from build123d import *

# Parameters (mm, degrees)
SKETCH1_R           = 5.75
SKETCH1_R_2         = 3
BOSS_EXTRUDE1_DEPTH = 6
SKETCH1_3_R         = 5.75
SKETCH1_3_R_2       = 3
BOSS_EXTRUDE2_DEPTH = 12


with BuildPart() as part:
    # Sketch1 → Boss-Extrude1 (new body)
    with BuildSketch(Plane.XY):
        Polygon((-3.464101615, 6), (-6.92820323, 0), (-3.464101615, -6), (3.464101615, -6), (6.92820323, 0), (3.464101615, 6), align=None)
        Circle(SKETCH1_R, mode=Mode.SUBTRACT)
        Circle(SKETCH1_R)
        Circle(SKETCH1_R_2, mode=Mode.SUBTRACT)
        Circle(SKETCH1_R_2)
    extrude(amount=BOSS_EXTRUDE1_DEPTH)

    # Sketch1_3 → Boss-Extrude2 (add)
    with BuildSketch(Plane.XY):
        Circle(SKETCH1_3_R)
        Circle(SKETCH1_3_R_2, mode=Mode.SUBTRACT)
    extrude(amount=-BOSS_EXTRUDE2_DEPTH)


solid = part.part
Input: part model. Units: mm. Frame: model coordinates. A direction names the side the tool comes from. Coordinates: 2 decimals unless noted, no trailing zeros. Loops run counter-clockwise (first coordinate to the right, second up) from the corner with the lowest first, then second, coordinate; pieces in that order, holes last. Notation, with made-up numbers: (65.25, 46) - (73.25, 46) arc R16 cw to (73.25, 62) - close; hole circle Ø5 at (26.5, 74.5). An arc over 180 degrees is marked (long way). Answer in a Markdown table with one row per item. Add a question column.
Item 1: Contact query for flat-ended pins moving along their axis: P1, Ø4, axis at y = -1.5, z = -7.5, coming from the -X side; P2, Ø1.5, axis at x = -2, z = -4, coming from the +Y side; P3, Ø1.5, axis at x = -4, z = -5, coming from the -Y side; P4, Ø5, axis at x = 0.5, y = -1, coming from the -Z side. Output: stop coordinate, or through.
Item 2: Section query B-B on x = 0. Return the cut outline in (y, z), then the cut area to 3 significant figures.
Item 3: Section query D-D on z = -1.5. Return the cut outline in (x, y), then the cut area to 3 significant figures.
Item 4: Section query C-C on y = 3.5. Return the cut outline in (x, z).
Item 5: Section query A-A on z = 2. Return the cut outline in (x, y).
Item 6: Mould query, pull axis X, two halves, no side actions, for faces 3 (the cylindrical face through (-3, 0, -6)), 4 (the flat face through (0, 0, 0)), 5 (the flat face through (0, -6, 3)), 6 (the flat face through (-5.22, -2.96, 2.96)). Classes: released by +X, released by -X, zero draft, split by the parting line, or undercut.
Item 7: Access query for faces 1 (the flat face through (6, 1, 0)), 2 (the flat face through (2.5, -2.5, -12)). Directions: +Z, -Z, +X, -X, +Y, -Y. A direction counts if a zero-diameter tool reaches every point of the face in a straight line with its end or side. Return the directions, or none.
Item 8: Line query: line 1 along Y through (x, z) = (0, -5.25); line 2 along Z through (x, y) = (1.5, 0.5); line 3 along Y through (x, z) = (2.5, -7.5). Output: solid intervals per line, ascending. Write a range as [from, to].
Recorded:
| question | item | result |
|---|---|---|
| 1 | P1 | x = -5.75 |
| 1 | P2 | y = 5.61 |
| 1 | P3 | y = -4.74 |
| 1 | P4 | z = -12 |
| 2 | outline | (-6, 0) - (-5.75, 0) - (-5.75, -12) - (-3, -12) - (-3, 0) - (3, 0) - (3, -12) - (5.75, -12) - (5.75, 0) - (6, 0) - (6, 6) - (-6, 6) - close |
| 2 | area | 138 mm^2 |
| 3 | outline | circle Ø11.5 at (0, 0); hole circle Ø6 at (0, 0) |
| 3 | area | 75.6 mm^2 |
| 4 | outline | (-4.91, 0) - (-4.56, 0) - (-4.56, -12) - (4.56, -12) - (4.56, 0) - (4.91, 0) - (4.91, 6) - (-4.91, 6) - close |
| 5 | outline | (-6.93, 0) - (-3.46, -6) - (3.46, -6) - (6.93, 0) - (3.46, 6) - (-3.46, 6) - close |
| 6 | face 3 | undercut |
| 6 | face 4 | undercut |
| 6 | face 5 | zero draft |
| 6 | face 6 | released by -X |
| 7 | face 1 | -Z |
| 7 | face 2 | -Z, +X, -X, +Y, -Y |
| 8 | line 1 | [-5.75, -3], [3, 5.75] |
| 8 | line 2 | [0, 6] |
| 8 | line 3 | [-5.18, -1.66], [1.66, 5.18] |
